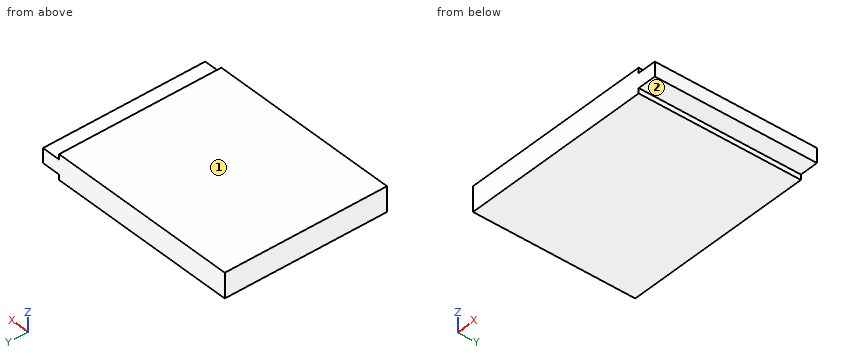
```python
from build123d import *

# Parameters (mm, degrees)
F0_W          = 61
F0_H          = 47
F1_DEPTH      = 7.18
F2_W          = 5.3985562474
F2_H          = 1.5
F3_DEPTH      = 23.501
F3_DEPTH_BACK = 23.501


with BuildPart() as f1:
    # F0 (on Top) → F1 (new body)
    with BuildSketch(Plane.XY):
        Rectangle(F0_W, F0_H)
    extrude(amount=F1_DEPTH)

    # F2 (on Front) → F3 (cut, two sides)
    with BuildSketch(Plane.XZ) as f3_sk:
        with Locations((27.8007218763, 0.75)):
            Rectangle(F2_W, F2_H)
        with Locations((27.8007218763, 6.43)):
            Rectangle(F2_W, F2_H)
    extrude(amount=-F3_DEPTH, mode=Mode.SUBTRACT)
    extrude(f3_sk.sketch, amount=F3_DEPTH_BACK, mode=Mode.SUBTRACT)


solid = f1.part
```
Verification items for the finished model (mm, model axes). Face numbers are marked on the shaded views. A direction names the side the tool comes from. Coordinates: 2 decimals unless noted, no trailing zeros. Write each loop counter-clockwise with the first axis right and the second up, starting at its lowest first coordinate (ties: lowest second). Pieces come first, ordered by that corner, then holes. Notation, with made-up numbers: M 74.5,38.5 L 115.5,38.5 A12 ccw 115.5,57.5 Z; hole C 24,23.5 d6. An arc over 180 degrees is marked long. Answer as a JSON object with one key per item and string values. Group by question number.
(1) Gauge pin test, flat ends, axial feed: pin 1 (6 mm diameter, centred on x = -10, y = 5, fed in from -Z); pin 2 (1.2 mm diameter, centred on y = 7.5, z = 0.5, fed in from +X); pin 3 (4.5 mm diameter, centred on x = 28, y = -11.5, fed in from -Z); pin 4 (1.6 mm diameter, centred on x = 29, y = 9, fed in from +Z). Record the tip position at first contact, or that the pin passes through.
(2) Cross-section at A-A, the plane y = -7.5. Record the cut outline in (x, z), and give its area (3 significant figures).
(3) Material ranges on line 1 (X direction, y = 20.5, z = 0.75), recorded low to high.
(4) Tool access check on the marked faces 1 and 2. Record the directions out of +Z, -Z, +X, -X, +Y, -Y that give a thin tool (end or side, any length) a straight path to the whole face; none if there is none.
Reply:
{
 "1": {"pin 1": "z = 0", "pin 2": "x = 25.1", "pin 3": "z = 1.5", "pin 4": "z = 5.68"},
 "2": {"outline": "M -30.5,0 L 25.1,0 L 25.1,1.5 L 30.5,1.5 L 30.5,5.68 L 25.1,5.68 L 25.1,7.18 L -30.5,7.18 Z", "area": "422 mm²"},
 "3": {"line 1": "-30.5 to 25.1"},
 "4": {"face 1": "+Z, +X, -X, +Y, -Y", "face 2": "-Z, +X, +Y, -Y"}
}
